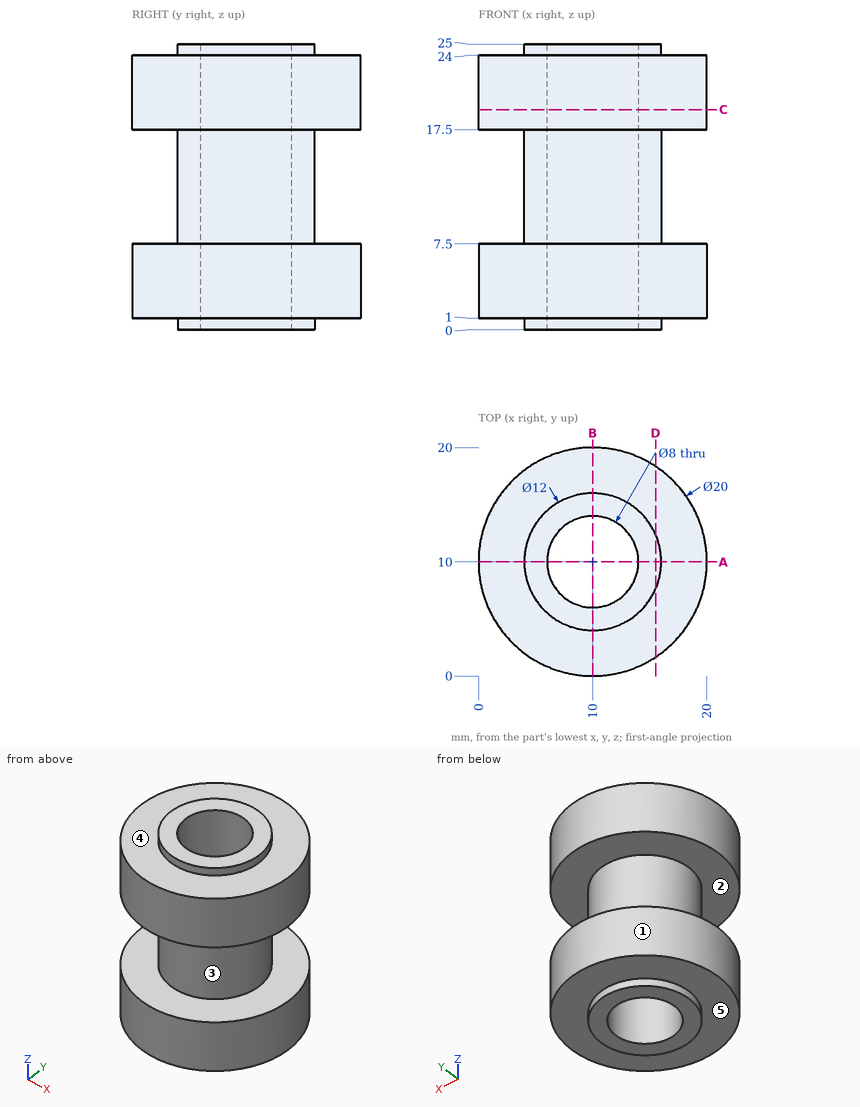
Here's the drawing with two shaded views (mm, measured from the low corner). I have some questions. A direction names the side the tool comes from. Round coordinates to 2 decimals unless told otherwise and drop trailing zeros. Write each loop counter-clockwise with the first axis right and the second up, starting at its lowest first coordinate (ties: lowest second). Pieces come first, ordered by that corner, then holes. Notation, with made-up numbers: M -9.5,11.5 L 46.5,11.5 A23 cw 46.5,48.5 Z; hole C 15.25,79 d10. An arc over 180 degrees is marked long. Write each question's results on one line, items separated by ' | '. Start each with the question number.
1. Imagine slicing it at D-D on x = 15.5. List the corners of the cut face in (y, z) for me, and give its area (3 significant figures).
2. Imagine slicing it at C-C on z = 19.25. List the corners of the cut face in (x, y) for me.
3. Thinking about a two-plate mould opening in Z: for the marked faces 3, 4 and 5, which applies, +Z half, -Z half, draft (parallel to the pull), parting line (faces both ways), or undercut?
4. I need wall thicknesses on L1, parallel to Z at x = 4, y = 15.75; L2, parallel to Y at x = 10, z = 19.5; L3, parallel to X at y = 9.75, z = 4.5. Which ranges of each line are inside material? Lowest first, please. Write a range as from..to.
5. I'm going to push flat-ended pins straight in: pin 1 Ø3 at (x, z) = (5, 12) entering from +Y; pin 2 Ø1.5 at (x, y) = (16.5, 14.5) entering from -Z; pin 3 Ø6 at (x, y) = (11, 11) entering from +Z. Where does each tip first touch, or does it pass through?
6. On a 3-axis mill with a long thin cutter (end or side, diameter ignored), from which of +Z, -Z, +X, -X, +Y, -Y can I reach the whole of each face in a straight line? I mean the marked faces 1 and 2. Say none if no direction works.
7. Imagine slicing it at A-A on y = 10. List the corners of the cut face in (x, z) for me.
Result sheet:
1) outline: M 1.65,1 L 7.6,1 L 7.6,0 L 12.4,0 L 12.4,1 L 18.35,1 L 18.35,7.5 L 12.4,7.5 L 12.4,17.5 L 18.35,17.5 L 18.35,24 L 12.4,24 L 12.4,25 L 7.6,25 L 7.6,24 L 1.65,24 L 1.65,17.5 L 7.6,17.5 L 7.6,7.5 L 1.65,7.5 Z | area: 275 mm^2
2) outline: C 10,10 d20; hole C 10,10 d8
3) face 3: undercut | face 4: +Z half | face 5: -Z half
4) L1: z = 1..7.5, 17.5..24 | L2: y = 0..6, 14..20 | L3: x = 0..6.01, 13.99..20
5) pin 1: stops at y = 14.87 | pin 2: stops at z = 1 | pin 3: stops at z = 25
6) face 1: +Z, -Z | face 2: none
7) outline: M 0,1 L 4,1 L 4,0 L 6,0 L 6,25 L 4,25 L 4,24 L 0,24 L 0,17.5 L 4,17.5 L 4,7.5 L 0,7.5 Z; M 14,0 L 16,0 L 16,1 L 20,1 L 20,7.5 L 16,7.5 L 16,17.5 L 20,17.5 L 20,24 L 16,24 L 16,25 L 14,25 Z
